Geometry check sheet. Reference: drawing and pictorial views, mm from the part's lowest x, y, z. A direction names the side the tool comes from. Round coordinates to 2 decimals unless told otherwise and drop trailing zeros. Write each loop counter-clockwise with the first axis right and the second up, starting at its lowest first coordinate (ties: lowest second). Pieces come first, ordered by that corner, then holes.
Item 1: Section check D-D, the plane y = 13.75. Record the cut outline in (x, z).
Item 2: Set-up check for the marked faces 4, 5, 6 and 7: record each of +Z, -Z, +X, -X, +Y, -Y from which the full face is reachable in a straight line by a thin tool's end or side.
Item 3: Section check B-B, the plane x = 17. Record the cut outline in (y, z), plus the area to 3 significant figures.
Item 4: Release check for a two-part mould opening along X. For the marked faces 1, 2 and 3 record: pulls with the +X half, pulls with the -X half, needs draft (parallel to the pull), parting line crosses it, or undercut.
Item 5: Material ranges on line 1 along Y through (x, z) = (17.5, 4.5); line 2 along X through (y, z) = (9, 0.35); line 3 along Y through (x, z) = (3.5, 1.85), recorded low to high.
Item 6: Depth check by flat-ended pin: pin 1 (2.5 mm diameter, centred on x = 27.5, z = 1.5, fed in from -Y); pin 2 (1 mm diameter, centred on y = 6, z = 1.5, fed in from -X); pin 3 (1.6 mm diameter, centred on x = 2.5, z = 3, fed in from -Y); pin 4 (1 mm diameter, centred on x = 14.5, y = 18, fed in from -Z). Enter the tip coordinate at first touch or a pass-through.
Item 7: Section check C-C, the plane z = 3.6. Record the cut outline in (x, y).
Item 8: Section check A-A, the plane y = 6.75. Record the cut outline in (x, z).
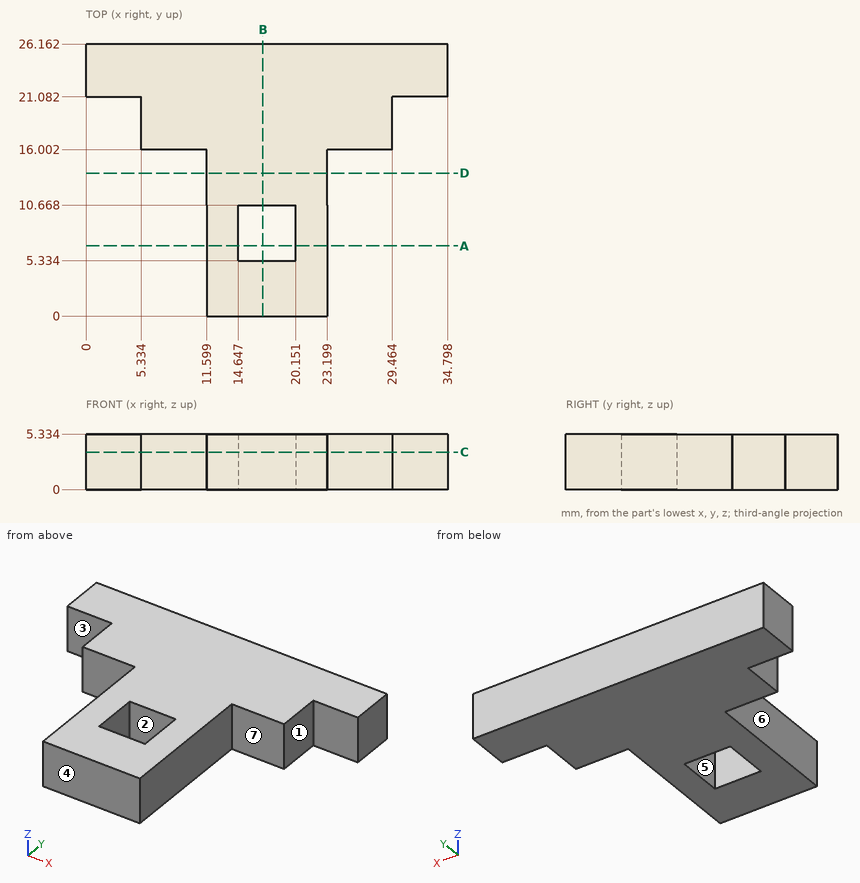
Values found:
1. outline: (11.6, 0) - (23.2, 0) - (23.2, 5.33) - (11.6, 5.33) - close
2. face 4: +Z, -Z, +X, -X, -Y
2. face 5: +Z, -Z
2. face 6: +Z, -Z, -X, -Y
2. face 7: +Z, -Z, +X, -Y
3. outline: (0, 0) - (5.33, 0) - (5.33, 5.33) - (0, 5.33) - close; (10.67, 0) - (26.16, 0) - (26.16, 5.33) - (10.67, 5.33) - close
3. area: 111 mm2
4. face 1: pulls with the +X half
4. face 2: undercut
4. face 3: needs draft
5. line 1: y = 0 to 5.33, 10.67 to 26.16
5. line 2: x = 11.6 to 14.65, 20.15 to 23.2
5. line 3: y = 21.08 to 26.16
6. pin 1: stops at y = 16
6. pin 2: stops at x = 11.6
6. pin 3: stops at y = 21.08
6. pin 4: stops at z = 0
7. outline: (0, 21.08) - (5.33, 21.08) - (5.33, 16) - (11.6, 16) - (11.6, 0) - (23.2, 0) - (23.2, 16) - (29.46, 16) - (29.46, 21.08) - (34.8, 21.08) - (34.8, 26.16) - (0, 26.16) - close; hole (14.65, 5.33) - (20.15, 5.33) - (20.15, 10.67) - (14.65, 10.67) - close
8. outline: (11.6, 0) - (14.65, 0) - (14.65, 5.33) - (11.6, 5.33) - close; (20.15, 0) - (23.2, 0) - (23.2, 5.33) - (20.15, 5.33) - close
